Source: CAD feature listing. Evaluate the final solid. Frame: model axes, mm. A direction names the side the tool comes from. Give positions to 0.01 mm unless a question says otherwise; leave off trailing zeros. Order: outer loops, then holes, each group sorted by start corner. A loop starts at its lowest first (then second) coordinate and runs counter-clockwise, first axis right, second up. Notation, with made-up numbers: M 22.25,41 L 35.25,41 A24 ccw 35.25,78 Z; hole C 76.5,-19 d3. An arc over 180 degrees is marked long. Use CSV: the item, a comma, the result in double quotes. Start each with the question number.
Item 1: Ray query, probe 1 along X at (y, z) = (17.5, 0.3); probe 2 along X at (y, z) = (20.5, 3.6); probe 3 along Y at (x, z) = (13, 0.85). Return the intervals inside material, ascending. Write a range as from..to.
Item 2: First-contact query: pin 1 (1.9 mm diameter, centred on y = 0, z = 1.5, fed in from +X); pin 2 (1 mm diameter, centred on x = 13, z = 3, fed in from +Y). Flat tips, straight axial feed; report the tip coordinate or a pass-through.
Item 3: Section query B-B on x = 2.5. Return loops of the section in (y, z), and give its area (3 significant figures).
Item 4: Access query for faces 1 (the face through (12.83, -14.63, 1.88)), 2 (the face through (1.983, 3.503, 1.878)). Directions: +Z, -Z, +X, -X, +Y, -Y. A direction counts if a zero-diameter tool reaches every point of the face in a straight line with its end or side. Return the directions, or none.
Item 5: Section query C-C on z = 1.8. Count the separate pieces of the cut face and the enclosed holes in it, and give its area (3 significant figures).
Item 6: Section query D-D on x = 17.5. Return loops of the section in (y, z), and give its area (3 significant figures).
Item 7: Section query A-A on y = -11. Return loops of the section in (x, z).
from build123d import *

# Parameters (mm, degrees)
F1_DEPTH = 3.81
F2_DEPTH = 25.4
F4_DEPTH = 25.4
F5_DEPTH = 25.4
F7_DEPTH = 25.4


with BuildPart() as f1:
    # F0 (on Top) → F1 (new body)
    with BuildSketch(Plane.XY):
        Polygon((6.5642443103, 3.7926732977), (-0.0024292689, 7.5811389783), (-6.5666735793, 3.7884656805), (-6.5642443103, -3.7926732977), (0.0024292689, -7.5811389783), (6.5666735793, -3.7884656805), align=None)
        Polygon((-4.0262038002, 2.3228099792), (-0.00148945, 4.6481997614), (4.0247143502, 2.3253897822), (4.0262038002, -2.3228099792), (0.00148945, -4.6481997614), (-4.0247143502, -2.3253897822), align=None, mode=Mode.SUBTRACT)
    extrude(amount=F1_DEPTH)

    # F2 (add): a face of the model
    f2_faces = [f1.faces().sort_by_distance(p)[0] for p in [
        (3.2845514241, -5.6848023294, 1.905),
    ]]
    extrude(f2_faces, amount=F2_DEPTH)

    # F3 (on face) → F4 (cut)
    with BuildSketch(Plane.XY.offset(3.81)):
        Polygon((3.4240530816, -9.5536917259), (9.0931520865, -16.0562525411), (9.3687364086, -15.8970260939), (6.5666733931, -7.7379561169), (4.9953633304, -8.6458238677), align=None)
        Polygon((9.9074144135, -17.4655531656), (12.7094772591, -25.6246232408), (14.2807875079, -24.7167553825), (10.0452065827, -17.3859399373), align=None)
        Polygon((10.0452065827, -17.3859399373), (14.2807875079, -24.7167553825), (15.8520975706, -23.8088876318), (10.1829987356, -17.3063267185), align=None)
    extrude(amount=-F4_DEPTH, mode=Mode.SUBTRACT)

    # F5 (add): a face of the model
    f5_faces = [f1.faces().sort_by_distance(p)[0] for p in [
        (-3.2845514241, 5.6848023294, 1.905),
    ]]
    extrude(f5_faces, amount=F5_DEPTH)

    # F6 (on face) → F7 (cut)
    with BuildSketch(Plane.XY.offset(3.81)):
        Polygon((6.5666733931, -7.7379561169), (3.4240530816, -9.5536917259), (9.0931520865, -16.0562525411), (9.3687364086, -15.8970260939), align=None)
        Polygon((12.7094772591, -25.6246232408), (15.8520975706, -23.8088876318), (10.1829987356, -17.3063267185), (9.9074144135, -17.4655531656), align=None)
        Polygon((-9.3687364249, 15.8970260845), (-6.5666735793, 7.7379560094), (-3.4240532678, 9.5536916184), (-9.0931521028, 16.0562525317), align=None)
        Polygon((-9.9074144298, 17.4655531562), (-12.7094774453, 25.6246231332), (-15.8520977568, 23.8088875242), (-10.1829987519, 17.306326709), align=None)
    extrude(amount=-F7_DEPTH, mode=Mode.SUBTRACT)


solid = f1.part
Verdict:
1,probe 1,"-14.49..-10.35, -9.92..-5.73"
1,probe 2,"-16.22..-12.97, -10.95..-7.47"
1,probe 3,"-29.41..-25.46, -20.54..-14.92"
2,pin 1,"x = 6.57"
2,pin 2,"y = -14.06"
3,outline,"M -11.9,0 L -3.2,0 L -3.2,3.81 L -11.9,3.81 Z; M 3.21,0 L 6.14,0 L 6.14,3.81 L 3.21,3.81 Z"
3,area,"44.3 mm2"
4,face 1,"+Z, -Z, +X, +Y"
4,face 2,"+Z, -Z"
5,separate pieces,"1"
5,enclosed holes,"5"
5,area,"411 mm2"
6,outline,"M -26.81,0 L -22.71,0 L -22.71,3.81 L -26.81,3.81 Z"
6,area,"15.6 mm2"
7,outline,"M 1.98,0 L 4.68,0 L 4.68,3.81 L 1.98,3.81 Z; M 7.69,0 L 10.73,0 L 10.73,3.81 L 7.69,3.81 Z"
